For this review, take the finished solid that the model builds, in its own axes (mm). Face numbers are marked on the shaded views. A direction names the side the tool comes from. Give positions to 0.01 mm unless a question says otherwise; leave off trailing zeros. Write each loop counter-clockwise with the first axis right and the second up, starting at its lowest first coordinate (ties: lowest second). Pieces come first, ordered by that corner, then holes.
1) We need section B-B on y = 0. Give the boundary of the cut face in (x, z).
2) We need section C-C on z = 5.5. Give the boundary of the cut face in (x, y), and give its area (3 significant figures).
3) Wall thickness on line 1 along X through (y, z) = (-13, 4.25); line 2 along X through (y, z) = (11.5, 1.75); line 3 along Y through (x, z) = (-12, 5.5): over which ranges is each line inside the solid? List them lowest first.
4) For P1, Ø0.8, axis at x = 9, z = 3.5, coming from the -Y side; P2, Ø5, axis at x = 11.5, z = 4.5, coming from the +Y side; P3, Ø1.5, axis at x = -16.5, z = 2, coming from the +Y side; P4, Ø4.5, axis at y = -0.5, z = 6, coming from the -X side, all flat-tipped, find the tip position at first contact; note any pin that passes through.
5) Draft analysis for pull direction Y (two halves, no side actions). For the marked faces 1, 2 and 3, state which applies: pulls with the +Y half, pulls with the -Y half, needs draft (parallel to the pull), parting line crosses it, or undercut.
6) We need section A-A on x = 0. Give the number of separate pieces and of enclosed holes in the cut face, and give its area (3 significant figures).
7) Machinability: for the marked faces 4 and 5, which of the approach directions +Z, -Z, +X, -X, +Y, -Y give a long, thin tool a straight path to every point of the face, cutting with its end or side? Answer none if there is none.
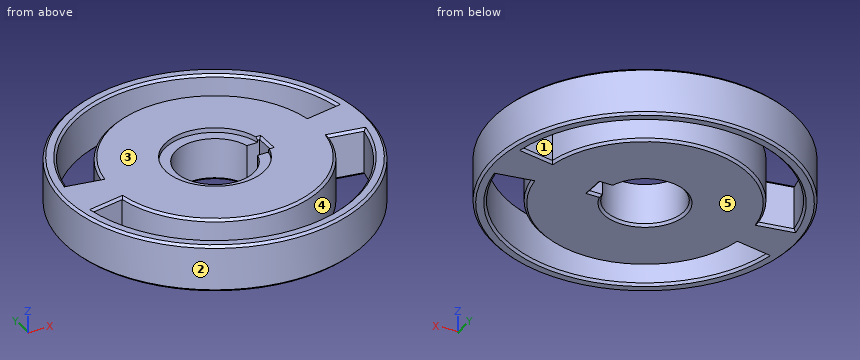
from build123d import *

# Parameters (mm, degrees)
SKETCH_1_R          = 32
EXTRUDE_1_DEPTH     = 10
SKETCH_2_R          = 8.25
CUT_EXTRUDE_1_DEPTH = 10
SKETCH_4_W          = 2.746324374
SKETCH_4_H          = 4.000918907
CUT_EXTRUDE_3_DEPTH = 10
CUT_EXTRUDE_4_DEPTH = 10
CUT_EXTRUDE_5_DEPTH = 10
CHAMFER_1_SIZE      = 0.5
CHAMFER_2_SIZE      = 0.5
SKETCH_7_R          = 10.5
CUT_EXTRUDE_6_DEPTH = 1


with BuildPart() as part:
    # 草图1 → 凸台-拉伸1 (new body)
    with BuildSketch(Plane.XY):
        Circle(SKETCH_1_R)
    extrude(amount=EXTRUDE_1_DEPTH)

    # 草图2 → 切除-拉伸1 (cut)
    with BuildSketch(Plane.XY):
        Circle(SKETCH_2_R)
    extrude(amount=CUT_EXTRUDE_1_DEPTH, mode=Mode.SUBTRACT)

    # 草图4 → 切除-拉伸3 (cut)
    with BuildSketch(Plane.XY):
        with Locations((9.376837813, -0.000459453)):
            Rectangle(SKETCH_4_W, SKETCH_4_H)
    extrude(amount=CUT_EXTRUDE_3_DEPTH, mode=Mode.SUBTRACT)

    # 草图5 → 切除-拉伸4 (cut)
    with BuildSketch(Plane.XY):
        with BuildLine():
            Line((-22.1582, 3.9071), (-29.0518, 5.1226))
            ThreePointArc((-29.0518, 5.1226), (0, 29.5), (29.0518, 5.1226))
            Line((29.0518, 5.1226), (22.1582, 3.9071))
            ThreePointArc((22.1582, 3.9071), (0, 22.5), (-22.1582, 3.9071))
        make_face()
    extrude(amount=CUT_EXTRUDE_4_DEPTH, mode=Mode.SUBTRACT)

    # 草图6 → 切除-拉伸5 (cut)
    with BuildSketch(Plane.XY):
        with BuildLine():
            Line((22.1582, -3.9071), (29.0518, -5.1226))
            ThreePointArc((29.0518, -5.1226), (0, -29.5), (-29.0518, -5.1226))
            Line((-29.0518, -5.1226), (-22.1582, -3.9071))
            ThreePointArc((-22.1582, -3.9071), (0, -22.5), (22.1582, -3.9071))
        make_face()
    extrude(amount=CUT_EXTRUDE_5_DEPTH, mode=Mode.SUBTRACT)

    # 倒角1
    chamfer_1_edges = [part.edges().sort_by_distance(p)[0] for p in [
        (9.376952648, 2, 10),
        (9.376837813, -2.000918907, 10),
        (10.75, -0.000459453, 10),
        (0, 22.5, 10),
        (25.605, 4.51485, 10),
        (0, 29.5, 10),
        (-25.605, 4.51485, 10),
        (0, -22.5, 10),
        (-32, 0, 10),
        (-25.605, -4.51485, 10),
        (0, -29.5, 10),
        (25.605, -4.51485, 10),
        (-8.249999986, 0.000473587, 10),
    ]]
    chamfer(chamfer_1_edges, length=CHAMFER_1_SIZE)

    # 倒角2
    chamfer_2_edges = [part.edges().sort_by_distance(p)[0] for p in [
        (9.376837813, -2.000918907, 0),
        (10.75, -0.000459453, 0),
        (9.376952648, 2, 0),
        (-32, 0, 0),
        (0, 22.5, 0),
        (25.605, 4.51485, 0),
        (0, 29.5, 0),
        (-25.605, 4.51485, 0),
        (0, -22.5, 0),
        (-25.605, -4.51485, 0),
        (0, -29.5, 0),
        (25.605, -4.51485, 0),
        (-8.249999986, 0.000473587, 0),
    ]]
    chamfer(chamfer_2_edges, length=CHAMFER_2_SIZE)

    # 草图7 → 切除-拉伸6 (cut)
    with BuildSketch(Plane.XY.offset(10)):
        Circle(SKETCH_7_R)
    extrude(amount=-CUT_EXTRUDE_6_DEPTH, mode=Mode.SUBTRACT)


solid = part.part
Results list:
1. outline: (-32, 0.5) - (-31.5, 0) - (-8.75, 0) - (-8.25, 0.5) - (-8.25, 9) - (-10.5, 9) - (-10.5, 10) - (-31.5, 10) - (-32, 9.5) - close; (10.75, 0.5) - (11.25, 0) - (31.5, 0) - (32, 0.5) - (32, 9.5) - (31.5, 10) - (11.25, 10) - (10.75, 9.5) - close
2. outline: circle Ø64 at (0, 0); hole (-29.05, -5.12) arc R29.5 ccw to (29.05, -5.12) - (22.16, -3.91) arc R22.5 cw to (-22.16, -3.91) - close; hole (-29.05, 5.12) - (-22.16, 3.91) arc R22.5 cw to (22.16, 3.91) - (29.05, 5.12) arc R29.5 ccw to start; hole (8, -2) - (10.75, -2) - (10.75, 2) - (8, 2) arc R8.25 ccw (long way) to start
2. area: 1,980 mm2
3. line 1: x = -29.24 to -26.48, -18.36 to 18.36, 26.48 to 29.24
3. line 2: x = -29.86 to -27.17, -19.34 to 19.34, 27.17 to 29.86
3. line 3: y = -29.66 to -26.95, -19.03 to 19.03, 26.95 to 29.66
4. P1: stops at y = -30.82
4. P2: stops at y = 30.71
4. P3: stops at y = 27.86
4. P4: stops at x = -32
5. face 1: undercut
5. face 2: parting line crosses it
5. face 3: needs draft
6. separate pieces: 4
6. enclosed holes: 0
6. area: 329 mm2
7. face 4: +Z, -Z
7. face 5: -Z, +X, -X, +Y, -Y
